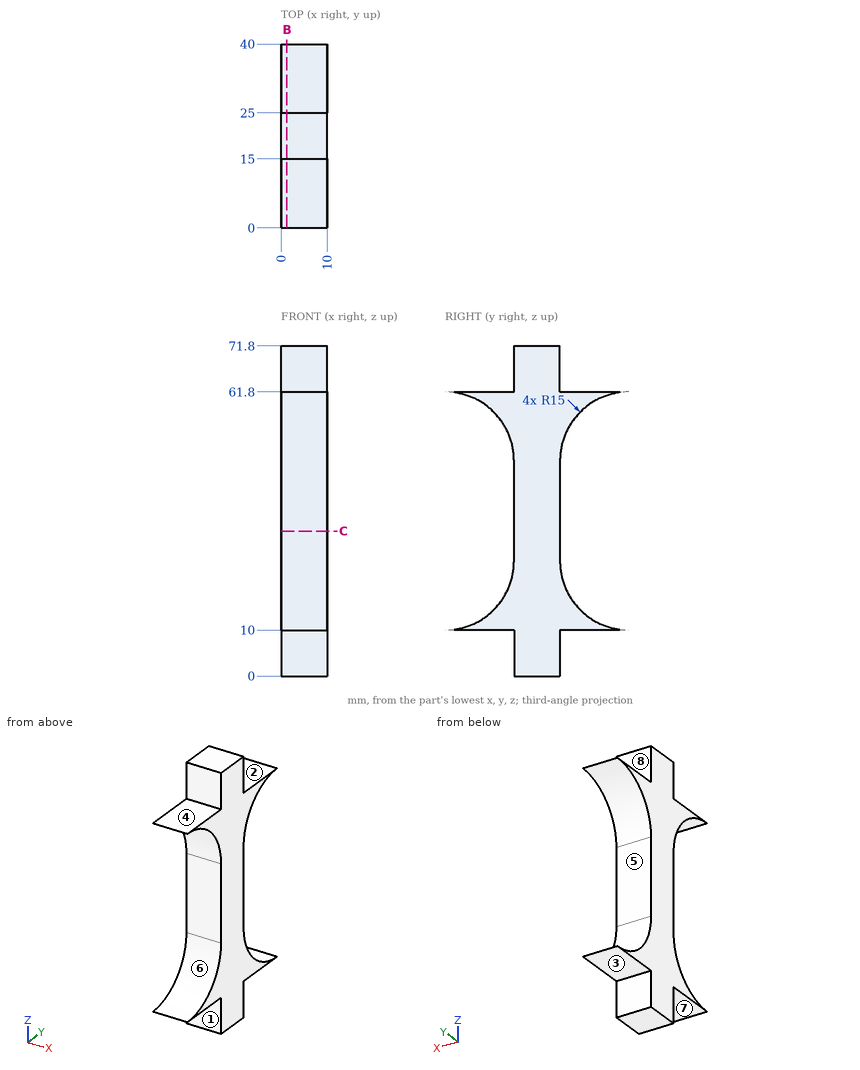
Answer from the drawing. Dimensions are ordinates in mm from the lowest x, y and z of the part. A direction names the side the tool comes from. Give positions to 0.01 mm unless a question says otherwise; leave off trailing zeros. Write each loop counter-clockwise with the first axis right and the second up, starting at its lowest first coordinate (ties: lowest second). Pieces come first, ordered by that corner, then holes. Notation, with made-up numbers: (7, 3.5) - (20, 3.5) arc R11 cw to (20, 17.5) - close; hole circle Ø8 at (38.25, 57). An arc over 180 degrees is marked (long way). One line per item, written item: value. Start each with the question number.
1. Find section B-B (x = 1.25). Write down the section's boundary in (y, z).
2. For the marked faces 1, 2, 3, 4 and 5, determine the directions among +Z, -Z, +X, -X, +Y, -Y from which every point of the face is accessible in a straight line to the end or side of a thin tool.
3. Consider probe 1 along Y at (x, z) = (6.25, 27.5); probe 2 along Z at (x, y) = (4, 36.5); probe 3 along Z at (x, y) = (4.25, 29.5). Determine where each line is inside the solid, lowest interval first.
4. Given pin 1 (3 mm diameter, centred on x = 4, z = 6, fed in from +Y); pin 2 (3 mm diameter, centred on x = 9, z = 29.5, fed in from -Y); pin 3 (3 mm diameter, centred on x = 3, y = 30.5, fed in from +Z), each flat-ended and moving along its own axis, determine where each tip first touches the part or whether it passes through.
5. For a pull along Z with two mould halves and no side action, classify the marked faces 6, 7 and 8 as +Z half, -Z half, draft (parallel to the pull), parting line (faces both ways), or undercut.
6. Find section C-C (z = 31.5). Write down the section's boundary in (x, y).
Geometry results:
1. outline: (0, 10) - (15, 10) - (15, 0) - (25, 0) - (25, 10) - (40, 10) arc R15 cw to (25, 25) - (25, 46.8) arc R15 cw to (40, 61.8) - (25, 61.8) - (25, 71.8) - (15, 71.8) - (15, 61.8) - (0, 61.8) arc R15 cw to (15, 46.8) - (15, 25) arc R15 cw to start
2. face 1: -Z, +X, -X, -Y
2. face 2: +Z, +X, -X, +Y
2. face 3: -Z, +X, -X, +Y
2. face 4: +Z, +X, -X, -Y
2. face 5: +X, -X, +Y
3. probe 1: 15 to 25
3. probe 2: 10 to 10.41, 61.39 to 61.8
3. probe 3: 10 to 14.29, 57.51 to 61.8
4. pin 1: y = 25
4. pin 2: y = 15
4. pin 3: z = 61.8
5. face 6: undercut
5. face 7: -Z half
5. face 8: draft
6. outline: (0, 15) - (10, 15) - (10, 25) - (0, 25) - close
